```python
from build123d import *

# Parameters (mm, degrees)
SKETCH1_R           = 3
BOSS_EXTRUDE1_DEPTH = 2


with BuildPart() as part:
    # Sketch1 → Boss-Extrude1 (new body)
    with BuildSketch(Plane.XY):
        Polygon((-142.75, 49.5), (-142.75, 0), (0, 0), (142.75, 0), (142.75, 49.5), align=None)
        with Locations((124.75, 30.5)):
            Circle(SKETCH1_R, mode=Mode.SUBTRACT)
        with Locations((75.25, 30.5)):
            Circle(SKETCH1_R, mode=Mode.SUBTRACT)
        with Locations((-75.25, 30.5)):
            Circle(SKETCH1_R, mode=Mode.SUBTRACT)
        with Locations((-124.75, 30.5)):
            Circle(SKETCH1_R, mode=Mode.SUBTRACT)
    extrude(amount=BOSS_EXTRUDE1_DEPTH)


solid = part.part
```
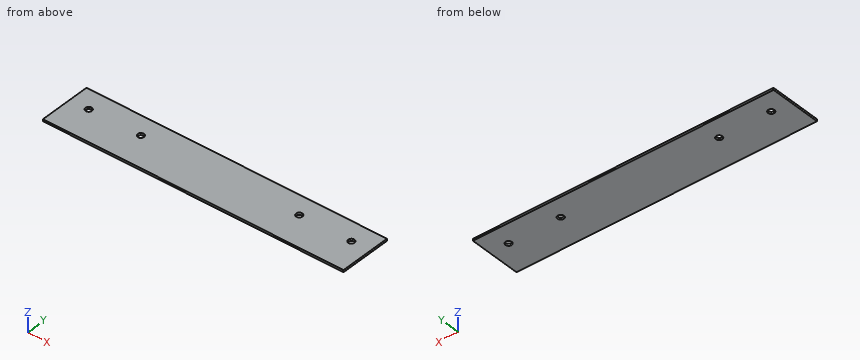
Can you work these out from the model? Positions are in its coordinate system, mm. Round coordinates to 2 decimals unless told otherwise and drop trailing zeros. Order: outer loops, then holes, each group sorted by start corner. A loop starts at its lowest first (then second) coordinate and runs counter-clockwise, first axis right, second up.
(1) If we section it at B-B (x = -124.75): Please give me the cut outline in (y, z), plus the area to 3 significant figures.
Results are:
outline: (0, 0) - (27.5, 0) - (27.5, 2) - (0, 2) - close; (33.5, 0) - (49.5, 0) - (49.5, 2) - (33.5, 2) - close
area: 87.0 mm2
(2) If I drill on L1, parallel to Y at x = -124.75, z = 1.15; L2, parallel to X at y = 31.5, z = 0.6; L3, parallel to Y at x = -78, z = 0.55, over which ranges is the centre line in solid material (lowest first)?
Results are:
L1: y = 0 to 27.5, 33.5 to 49.5
L2: x = -142.75 to -127.58, -121.92 to -78.08, -72.42 to 72.42, 78.08 to 121.92, 127.58 to 142.75
L3: y = 0 to 29.3, 31.7 to 49.5
(3) If we section it at A-A (y = 30.5): Please give me the cut outline in (x, z).
Results are:
outline: (-142.75, 0) - (-127.75, 0) - (-127.75, 2) - (-142.75, 2) - close; (-121.75, 0) - (-78.25, 0) - (-78.25, 2) - (-121.75, 2) - close; (-72.25, 0) - (72.25, 0) - (72.25, 2) - (-72.25, 2) - close; (78.25, 0) - (121.75, 0) - (121.75, 2) - (78.25, 2) - close; (127.75, 0) - (142.75, 0) - (142.75, 2) - (127.75, 2) - close
(4) I'm going to push a flat-ended pin straight in: pin 1 (5.5 mm diameter, centred on x = 124.75, y = 30.5, fed in from +Z). Where does the tip first touch, or does it pass through?
Results are:
pin 1: passes through
